from build123d import *

# Parameters (mm, degrees)
SKETCH1_R           = 1.5
SKETCH1_R_2         = 8
SKETCH1_R_3         = 1.55
SKETCH1_R_4         = 2
SKETCH1_W           = 10
SKETCH1_H           = 5
BOSS_EXTRUDE1_DEPTH = 5
FILLET2_R           = 7
FILLET3_R           = 3
CUT_EXTRUDE1_DEPTH  = 6
FILLET4_R           = 6


with BuildPart() as part:
    # Sketch1 → Boss-Extrude1 (new body)
    with BuildSketch(Plane.XY):
        with BuildLine():
            Line((310, 43.5), (251, 43.5))
            Line((251, 43.5), (251, 39.5))
            Line((251, 39.5), (236.5, 39.5))
            Line((236.5, 39.5), (236.5, 43.5))
            Line((236.5, 43.5), (192.25, 43.5))
            Line((192.25, 43.5), (192.25, 39.5))
            Line((192.25, 39.5), (177.75, 39.5))
            Line((177.75, 39.5), (177.75, 43.5))
            Line((177.75, 43.5), (133.5, 43.5))
            Line((133.5, 43.5), (133.5, 39.5))
            Line((133.5, 39.5), (119, 39.5))
            Line((119, 39.5), (119, 43.5))
            Line((119, 43.5), (80.5, 43.5))
            Line((80.5, 43.5), (80.5, 39.5))
            Line((80.5, 39.5), (76.5, 39.5))
            Line((76.5, 39.5), (76.5, 43.5))
            Line((76.5, 43.5), (-6.5, 43.5))
            Line((-6.5, 43.5), (-30, 20))
            Line((-30, 20), (-30, 7.325414703))
            ThreePointArc((-30, 7.325414703), (-30.985037822, 4.947323034), (-33.36312949, 3.962285212))
            ThreePointArc((-33.36312949, 3.962285212), (-37.325414703, 0), (-33.36312949, -3.962285212))
            ThreePointArc((-33.36312949, -3.962285212), (-31.543016926, -4.324328111), (-30, -5.355339059))
            Line((-30, -5.355339059), (-14, -21.355339059))
            Line((-14, -21.355339059), (-14, -32))
            Line((-14, -32), (-6.5, -32))
            Line((-6.5, -32), (-6.5, -65))
            Line((-6.5, -65), (24.5, -65))
            Line((24.5, -65), (24.5, -35))
            Line((24.5, -35), (18.5, -35))
            Line((18.5, -35), (18.5, -4.6))
            Line((18.5, -4.6), (316.5, -4.6))
            Line((316.5, -4.6), (316.5, -20))
            Line((316.5, -20), (333, -20))
            Line((333, -20), (333, -2.3))
            Line((333, -2.3), (327, -2.3))
            ThreePointArc((327, -2.3), (324, 0.7), (327, 3.7))
            Line((327, 3.7), (333, 3.7))
            Line((333, 3.7), (333, 6.7))
            Line((333, 6.7), (337, 6.7))
            Line((337, 6.7), (337, 16.5))
            ThreePointArc((337, 16.5), (329.091883092, 35.591883092), (310, 43.5))
        make_face()
        with Locations((21.920310217, 0)):
            Circle(SKETCH1_R, mode=Mode.SUBTRACT)
        with Locations((-21.920310217, 0)):
            Circle(SKETCH1_R, mode=Mode.SUBTRACT)
        Circle(SKETCH1_R_2, mode=Mode.SUBTRACT)
        with Locations((-3.05, 37)):
            Circle(SKETCH1_R_3, mode=Mode.SUBTRACT)
        with Locations((22.05, 20)):
            Circle(SKETCH1_R_3, mode=Mode.SUBTRACT)
        with Locations((-3.05, -41.5)):
            Circle(SKETCH1_R_3, mode=Mode.SUBTRACT)
        with Locations((22.05, -58.5)):
            Circle(SKETCH1_R_3, mode=Mode.SUBTRACT)
        with Locations((72.5, 20.1)):
            Circle(SKETCH1_R_3, mode=Mode.SUBTRACT)
        with Locations((84.5, 12.5)):
            Circle(SKETCH1_R_3, mode=Mode.SUBTRACT)
        with Locations((-10.5, -27.55)):
            Circle(SKETCH1_R_3, mode=Mode.SUBTRACT)
        with Locations((14, -27.55)):
            Circle(SKETCH1_R_3, mode=Mode.SUBTRACT)
        with Locations((-33.36312949, 0)):
            Circle(SKETCH1_R, mode=Mode.SUBTRACT)
        with Locations((78.5, 27.751425951)):
            Circle(SKETCH1_R_4, mode=Mode.SUBTRACT)
        with Locations((22.5, 12.5)):
            Rectangle(SKETCH1_W, SKETCH1_H, mode=Mode.SUBTRACT)
        with Locations((152, 12.5)):
            Rectangle(SKETCH1_W, SKETCH1_H, mode=Mode.SUBTRACT)
        with Locations((308, 12.5)):
            Rectangle(SKETCH1_W, SKETCH1_H, mode=Mode.SUBTRACT)
        Polygon((58.427680349, 8), (61.427680349, 8), (61.427680349, 6.806102344), (66.427680349, 6.806102344), (66.427680349, 8), (76, 8), (76, 17), (66.427680349, 17), (66.427680349, 18.193897656), (61.427680349, 18.193897656), (61.427680349, 17), (58.427680349, 17), align=None, mode=Mode.SUBTRACT)
    extrude(amount=BOSS_EXTRUDE1_DEPTH)

    # Fillet2
    fillet2_edges = [part.edges().sort_by_distance(p)[0] for p in [
        (18.5, -4.6, 2.5),
    ]]
    fillet(fillet2_edges, radius=FILLET2_R)

    # Fillet3
    fillet3_edges = [part.edges().sort_by_distance(p)[0] for p in [
        (18.5, -35, 2.5),
    ]]
    fillet(fillet3_edges, radius=FILLET3_R)

    # Sketch2 → Cut-Extrude1 (cut, through all)
    with BuildSketch(Plane.XY.offset(5)):
        with BuildLine():
            Line((21.920310217, -1.5), (16.920310217, -1.5))
            ThreePointArc((16.920310217, -1.5), (15.420310217, 0), (16.920310217, 1.5))
            Line((16.920310217, 1.5), (21.920310217, 1.5))
            ThreePointArc((21.920310217, 1.5), (23.420310217, 0), (21.920310217, -1.5))
        make_face()
        with BuildLine():
            Line((0, -8), (-5, -8))
            ThreePointArc((-5, -8), (-13, 0), (-5, 8))
            Line((-5, 8), (0, 8))
            ThreePointArc((0, 8), (8, 0), (0, -8))
        make_face()
        with BuildLine():
            Line((-21.920310217, -1.5), (-26.920310217, -1.5))
            ThreePointArc((-26.920310217, -1.5), (-28.420310217, 0), (-26.920310217, 1.5))
            Line((-26.920310217, 1.5), (-21.920310217, 1.5))
            ThreePointArc((-21.920310217, 1.5), (-20.420310217, 0), (-21.920310217, -1.5))
        make_face()
    extrude(amount=-CUT_EXTRUDE1_DEPTH, mode=Mode.SUBTRACT)

    # Fillet4
    fillet4_edges = [part.edges().sort_by_distance(p)[0] for p in [
        (316.5, -4.6, 2.5),
    ]]
    fillet(fillet4_edges, radius=FILLET4_R)


solid = part.part
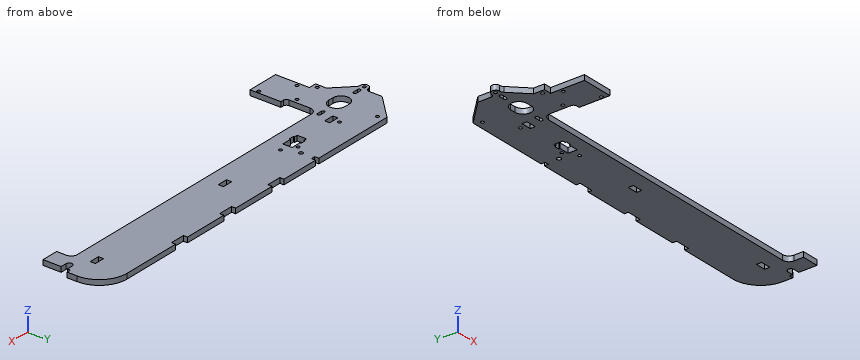
Could you check a few things on this model? Use its own coordinates, in mm. Coordinates: 2 decimals unless noted, no trailing zeros. Loops run counter-clockwise (first coordinate to the right, second up) from the corner with the lowest first, then second, coordinate; pieces in that order, holes last.
1. For P1, Ø1.5, axis at x = 328.5, z = 2, coming from the -Y side; P2, Ø0.6, axis at y = 17.5, z = 3, coming from the -X side; P3, Ø1.5, axis at x = -23.5, z = 3, coming from the +Y side, each with a flat end and sliding along its axis, tell me the tip position at first contact or that it passes through.
2. Imagine slicing it at A-A (x = 101). Please give me the cut outline in (y, z), and give its area (4 significant figures).
3. Imagine slicing it at B-B (y = -48). Please give me the cut outline in (x, z), and give its area (3 significant figures).
4. Imagine slicing it at C-C (z = 1.6). Give the number of separate pieces and of enclosed holes in the cut face, and give its area (3 significant figures).
5. I need wall thicknesses on L1, parallel to Y at x = 72.5, z = 3.95; L2, parallel to X at y = 15.5, z = 0.8; L3, parallel to Y at x = 307, z = 3.35. Which ranges of each line are inside material? Lowest first, please.
Computed values:
1. P1: stops at y = -20
1. P2: stops at x = -30
1. P3: stops at y = 27.25
2. outline: (-4.6, 0) - (43.5, 0) - (43.5, 5) - (-4.6, 5) - close
2. area: 240.5 mm2
3. outline: (-6.5, 0) - (24.5, 0) - (24.5, 5) - (-6.5, 5) - close
3. area: 155 mm2
4. separate pieces: 1
4. enclosed holes: 17
4. area: 18,600 mm2
5. L1: y = -4.6 to 8, 17 to 18.55, 21.65 to 43.5
5. L2: x = -30 to 58.43, 76 to 337
5. L3: y = -4.6 to 10, 15 to 43.5
